```python
from build123d import *

# Parameters (mm, degrees)
F1_DEPTH = 10
F2_R     = 5.5
F3_DEPTH = 0.5
F4_R     = 4
F5_DEPTH = 15


with BuildPart() as f1:
    # F0 (on Top) → F1 (new body)
    with BuildSketch(Plane.XY):
        Polygon((3.464102, 6), (-3.464102, 6), (-6.928203, 0), (-3.464102, -6), (3.464102, -6), (6.928203, 0), align=None)
    extrude(amount=F1_DEPTH)

    # F2 (on face) → F3 (join)
    with BuildSketch(Plane.XY.offset(10)):
        Circle(F2_R)
    extrude(amount=F3_DEPTH)

    # F4 (on face) → F5 (join)
    with BuildSketch(Plane.XY.offset(10.5)):
        Circle(F4_R)
    extrude(amount=F5_DEPTH)


solid = f1.part
```
Check sheet for the modelled part. Datum: model origin and axes. Units: mm. A direction names the side the tool comes from. Round coordinates to 2 decimals unless told otherwise and drop trailing zeros. Loops run counter-clockwise (first coordinate to the right, second up) from the corner with the lowest first, then second, coordinate; pieces in that order, holes last. Notation, with made-up numbers: (-15, 89.25) -> (37, 89.25) arc R30 cw to (37, 121.25) -> close; hole circle Ø3 at (55.25, 32.25). An arc over 180 degrees is marked (long way). Answer in a Markdown table with one row per item.
Q1. Set-up check for faces 1 (the face through (0, 0, 25.5)), 2 (the face through (-0.867, -3.905, 17.895)): record each of +Z, -Z, +X, -X, +Y, -Y from which the full face is reachable in a straight line by a thin tool's end or side.
Data:
| item | result |
|---|---|
| face 1 | +Z, +X, -X, +Y, -Y |
| face 2 | +Z |
Q2. Sectioned sample at A-A on x = 0. Enter the section's corners in (y, z), then the cut area to 4 significant figures.
Data:
| item | result |
|---|---|
| outline | (-6, 0) -> (6, 0) -> (6, 10) -> (5.5, 10) -> (5.5, 10.5) -> (4, 10.5) -> (4, 25.5) -> (-4, 25.5) -> (-4, 10.5) -> (-5.5, 10.5) -> (-5.5, 10) -> (-6, 10) -> close |
| area | 245.5 mm^2 |
Q3. Sectioned sample at D-D on x = -5. Enter the section's corners in (y, z), then the cut area to 3 significant figures.
Data:
| item | result |
|---|---|
| outline | (-3.34, 0) -> (3.34, 0) -> (3.34, 10) -> (2.29, 10) -> (2.29, 10.5) -> (-2.29, 10.5) -> (-2.29, 10) -> (-3.34, 10) -> close |
| area | 69.1 mm^2 |
Q4. Thickness scan on L1, parallel to Z at x = -3.75, y = -5; L2, parallel to Z at x = 4, y = -2.5; L3, parallel to Y at x = 0, z = 11.25. Record the ranges inside material, lowest first.
Data:
| item | result |
|---|---|
| L1 | z = 0 to 10 |
| L2 | z = 0 to 10.5 |
| L3 | y = -4 to 4 |
Q5. Sectioned sample at C-C on z = 11.25. Enter the section's corners in (x, y), then the cut area to 3 significant figures.
Data:
| item | result |
|---|---|
| outline | circle Ø8 at (0, 0) |
| area | 50.3 mm^2 |
Q6. Sectioned sample at B-B on y = -1.5. Enter the section's corners in (x, z).
Data:
| item | result |
|---|---|
| outline | (-6.06, 0) -> (6.06, 0) -> (6.06, 10) -> (5.29, 10) -> (5.29, 10.5) -> (3.71, 10.5) -> (3.71, 25.5) -> (-3.71, 25.5) -> (-3.71, 10.5) -> (-5.29, 10.5) -> (-5.29, 10) -> (-6.06, 10) -> close |
Q7. Go/stop test with flat-tipped pins: P1, Ø4, axis at x = -5, z = 14, coming from the -Y side; P2, Ø1, axis at x = 1, z = 18, coming from the +Y side; P3, Ø1.5, axis at y = -2.5, z = 13, coming from the +X side. Record where each tip stops, or that it passes through.
Data:
| item | result |
|---|---|
| P1 | stops at y = -2.65 |
| P2 | stops at y = 3.97 |
| P3 | stops at x = 3.6 |
